Read the model definition and answer for the solid it produces. Units are mm, in the model's axes. Face numbers are marked on the shaded views. A direction names the side the tool comes from. Coordinates: 2 decimals unless noted, no trailing zeros. Order: outer loops, then holes, each group sorted by start corner. A loop starts at its lowest first (then second) coordinate and runs counter-clockwise, first axis right, second up. Notation, with made-up numbers: (-15.75, 52) - (32.25, 52) arc R21 ccw to (32.25, 76) - close; hole circle Ø4 at (41, 38.5). An arc over 180 degrees is marked (long way). Use one line per item in the form item = value. Start each with the question number.
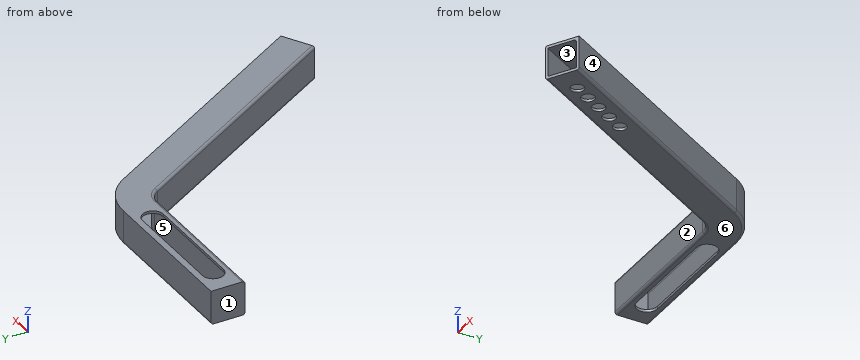
from build123d import *

# Parameters (mm, degrees)
BOSS_EXTRUDE1_DEPTH = 33.02
SHELL1_T            = -2.54
CUT_EXTRUDE1_REACH  = 409.111
SKETCH2_W           = 27.94
SKETCH2_H           = 27.94
CUT_EXTRUDE2_DEPTH  = 2.54
CUT_EXTRUDE3_REACH  = 303.28
CUT_EXTRUDE4_REACH  = 303.28
SKETCH6_R           = 6.35
CUT_EXTRUDE5_REACH  = 303.28
SKETCH7_R           = 6.35
SKETCH8_W           = 27.94
SKETCH8_H           = 27.94
BOSS_EXTRUDE2_DEPTH = 2.54
FILLET1_R           = 2.54


with BuildPart() as part:
    # Sketch1 → Boss-Extrude1 (new body)
    with BuildSketch(Plane.XY):
        with BuildLine():
            Line((-172.046968374, 25.4), (-23.576362049, 25.4))
            ThreePointArc((-23.576362049, 25.4), (1.823637951, 18.594090512), (20.417728463, 0))
            Line((20.417728463, 0), (152.4, -228.6))
            Line((152.4, -228.6), (123.803841167, -245.11))
            Line((123.803841167, -245.11), (-8.17843037, -16.51))
            ThreePointArc((-8.17843037, -16.51), (-14.686362049, -10.002068321), (-23.576362049, -7.62))
            Line((-23.576362049, -7.62), (-172.046968374, -7.62))
            Line((-172.046968374, -7.62), (-172.046968374, 25.4))
        make_face()
    extrude(amount=BOSS_EXTRUDE1_DEPTH)

    # Shell1
    shell1_openings = [part.faces().sort_by_distance(p)[0] for p in [
        (-172.046968374, 8.89, 16.51),
    ]]
    offset(amount=SHELL1_T, openings=shell1_openings, kind=Kind.INTERSECTION)

    # Sketch2 → Cut-Extrude1 (cut, up to next)
    with BuildSketch(Plane(origin=(137.086703653, -237.441135768, 0), x_dir=(0.8660254037844406, 0.4999999999999967, 0), z_dir=(0.4999999999999967, -0.8660254037844406, 0)), mode=Mode.PRIVATE) as cut_extrude1_sk1:
        with Locations((1.172271537, 16.51)):
            Rectangle(SKETCH2_W, SKETCH2_H)
    cut_extrude1_tool1 = extrude(cut_extrude1_sk1.sketch, amount=-CUT_EXTRUDE1_REACH, mode=Mode.PRIVATE) & part.part
    add(cut_extrude1_tool1.solids().sort_by_distance((138.101921, -236.855, 16.51))[0], mode=Mode.SUBTRACT)

    # Sketch3 → Cut-Extrude2 (cut)
    with BuildSketch(Plane.XY.offset(33.02)):
        with BuildLine():
            Line((-146.646968374, 19.05), (-45.046968374, 19.05))
            ThreePointArc((-45.046968374, 19.05), (-34.886968374, 8.89), (-45.046968374, -1.27))
            Line((-45.046968374, -1.27), (-50.126968374, -1.27))
            Line((-50.126968374, -1.27), (-146.646968374, -1.27))
            ThreePointArc((-146.646968374, -1.27), (-156.806968374, 8.89), (-146.646968374, 19.05))
        make_face()
    extrude(amount=-CUT_EXTRUDE2_DEPTH, mode=Mode.SUBTRACT)

    # Sketch4 → Cut-Extrude3 (cut, up to next)
    with BuildSketch(Plane(origin=(0, 0, 0), x_dir=(-1, 0, 0), z_dir=(0, 0, -1)), mode=Mode.PRIVATE) as cut_extrude3_sk1:
        with BuildLine():
            Line((45.046968374, -1.27), (146.646968374, -1.27))
            ThreePointArc((146.646968374, -1.27), (156.806968374, 8.89), (146.646968374, 19.05))
            Line((146.646968374, 19.05), (45.046968374, 19.05))
            ThreePointArc((45.046968374, 19.05), (34.886968374, 8.89), (45.046968374, -1.27))
        make_face()
    cut_extrude3_tool1 = extrude(cut_extrude3_sk1.sketch, amount=-CUT_EXTRUDE3_REACH, mode=Mode.PRIVATE) & part.part
    add(cut_extrude3_tool1.solids().sort_by_distance((-95.846968, 8.89, 0))[0], mode=Mode.SUBTRACT)

    # Sketch6 → Cut-Extrude4 (cut, up to next)
    with BuildSketch(Plane(origin=(0, 0, 0), x_dir=(-1, 0, 0), z_dir=(0, 0, -1)), mode=Mode.PRIVATE) as cut_extrude4_sk1:
        with Locations((-116.511920584, -199.460023065)):
            Circle(SKETCH6_R)
    cut_extrude4_tool1 = extrude(cut_extrude4_sk1.sketch, amount=-CUT_EXTRUDE4_REACH, mode=Mode.PRIVATE) & part.part
    # Sketch6 → Cut-Extrude4 (cut, up to next)
    with BuildSketch(Plane(origin=(0, 0, 0), x_dir=(-1, 0, 0), z_dir=(0, 0, -1)), mode=Mode.PRIVATE) as cut_extrude4_sk2:
        with Locations((-107.621920584, -184.062091385)):
            Circle(SKETCH6_R)
    cut_extrude4_tool2 = extrude(cut_extrude4_sk2.sketch, amount=-CUT_EXTRUDE4_REACH, mode=Mode.PRIVATE) & part.part
    # Sketch6 → Cut-Extrude4 (cut, up to next)
    with BuildSketch(Plane(origin=(0, 0, 0), x_dir=(-1, 0, 0), z_dir=(0, 0, -1)), mode=Mode.PRIVATE) as cut_extrude4_sk3:
        with Locations((-98.731920584, -168.664159706)):
            Circle(SKETCH6_R)
    cut_extrude4_tool3 = extrude(cut_extrude4_sk3.sketch, amount=-CUT_EXTRUDE4_REACH, mode=Mode.PRIVATE) & part.part
    # Sketch6 → Cut-Extrude4 (cut, up to next)
    with BuildSketch(Plane(origin=(0, 0, 0), x_dir=(-1, 0, 0), z_dir=(0, 0, -1)), mode=Mode.PRIVATE) as cut_extrude4_sk4:
        with Locations((-89.841920584, -153.266228027)):
            Circle(SKETCH6_R)
    cut_extrude4_tool4 = extrude(cut_extrude4_sk4.sketch, amount=-CUT_EXTRUDE4_REACH, mode=Mode.PRIVATE) & part.part
    add(cut_extrude4_tool1.solids().sort_by_distance((116.511921, -199.460023, 0))[0], mode=Mode.SUBTRACT)
    add(cut_extrude4_tool2.solids().sort_by_distance((107.621921, -184.062091, 0))[0], mode=Mode.SUBTRACT)
    add(cut_extrude4_tool3.solids().sort_by_distance((98.731921, -168.66416, 0))[0], mode=Mode.SUBTRACT)
    add(cut_extrude4_tool4.solids().sort_by_distance((89.841921, -153.266228, 0))[0], mode=Mode.SUBTRACT)

    # Sketch7 → Cut-Extrude5 (cut, up to next)
    with BuildSketch(Plane(origin=(0, 0, 0), x_dir=(-1, 0, 0), z_dir=(0, 0, -1)), mode=Mode.PRIVATE) as cut_extrude5_sk1:
        with Locations((-125.401920584, -214.857954744)):
            Circle(SKETCH7_R)
    cut_extrude5_tool1 = extrude(cut_extrude5_sk1.sketch, amount=-CUT_EXTRUDE5_REACH, mode=Mode.PRIVATE) & part.part
    add(cut_extrude5_tool1.solids().sort_by_distance((125.401921, -214.857955, 0))[0], mode=Mode.SUBTRACT)

    # Sketch8 → Boss-Extrude2 (add)
    with BuildSketch(Plane.ZY.offset(172.046968374)):
        with Locations((16.51, 8.89)):
            Rectangle(SKETCH8_W, SKETCH8_H)
    extrude(amount=-BOSS_EXTRUDE2_DEPTH)

    # Fillet1
    fillet1_edges = [part.edges().sort_by_distance(p)[0] for p in [
        (57.812705399, -130.81, 0),
        (-14.686362049, -10.002068321, 0),
        (-97.811665212, -7.62, 0),
        (-14.686362049, -10.002068321, 33.02),
        (57.812705399, -130.81, 33.02),
        (84.209159706, -115.57, 30.48),
        (0.553637951, 16.394385987, 30.48),
        (-96.541665212, 22.86, 30.48),
        (-97.811665212, 25.4, 0),
        (-97.811665212, -7.62, 33.02),
        (1.823637951, 18.594090512, 0),
        (86.408864232, -114.3, 0),
    ]]
    fillet(fillet1_edges, radius=FILLET1_R)


solid = part.part
Q1. For a pull along Y with two mould halves and no side action, classify the marked faces 3, 4, 5 and 6 as +Y half, -Y half, draft (parallel to the pull), parting line (faces both ways), or undercut.
Q2. Given P1, Ø10, axis at x = -100.5, z = 12, coming from the -Y side; P2, Ø0.8, axis at x = -90, z = 0.5, coming from the +Y side; P3, Ø2, axis at y = -137, z = 5, coming from the -X side; P4, Ø16.5, axis at x = 125.4, y = -214.86, coming from the -Z side, each flat-ended and moving along its own axis, determine where each tip first touches the part or whether it passes through.
Q3. A cutting plane is placed at B-B (z = 14.5). Give the vertices of the cut face in (x, y).
Q4. Consider probe 1 along Y at (x, z) = (-42.5, 6.5); probe 2 along Z at (x, y) = (118, -222.5); probe 3 along Y at (x, z) = (61, 27). Determine where each line is inside the solid, lowest interval first.
Q5. Which of the six approach directions +Z, -Z, +X, -X, +Y, -Y give full straight-line access (tool end or side, diameter ignored) to the marked faces 1 and 2?
Q6. A cutting plane is placed at A-A (x = -62.5). Give the vertices of the cut face in (y, z).
Result sheet:
q1.face_3 = undercut
q1.face_4 = +Y half
q1.face_5 = undercut
q1.face_6 = draft
q2.P1 = -7.62
q2.P2 = 24.8
q2.P3 = 60.81
q2.P4 = 0
q3.outline = (-172.05, -7.62) - (-23.58, -7.62) arc R17.78 cw to (-8.18, -16.51) - (123.8, -245.11) - (126, -243.84) - (-5.98, -15.24) arc R20.32 ccw to (-23.58, -5.08) - (-169.51, -5.08) - (-169.51, 22.86) - (-23.58, 22.86) arc R48.26 cw to (18.22, -1.27) - (150.2, -229.87) - (152.4, -228.6) - (20.42, 0) arc R50.8 ccw to (-23.58, 25.4) - (-172.05, 25.4) - close
q4.probe_1 = -7.62 to -5.08, 22.86 to 25.4
q4.probe_2 = 0 to 2.54, 30.48 to 33.02
q4.probe_3 = -136.33 to -131.25, -75.37 to -70.29
q5.face_1 = +Z, -Z, -X, +Y, -Y
q5.face_2 = +Z, -Z, -X, -Y
q6.outline = (-7.62, 2.54) arc R2.54 ccw to (-5.08, 0) - (-1.27, 0) - (-1.27, 2.54) - (-5.08, 2.54) - (-5.08, 30.48) - (-1.27, 30.48) - (-1.27, 33.02) - (-5.08, 33.02) arc R2.54 ccw to (-7.62, 30.48) - close; (19.05, 0) - (22.86, 0) arc R2.54 ccw to (25.4, 2.54) - (25.4, 33.02) - (19.05, 33.02) - (19.05, 30.48) - (20.32, 30.48) arc R2.54 cw to (22.86, 27.94) - (22.86, 2.54) - (19.05, 2.54) - close
